from build123d import *

# Parameters (mm, degrees)
F0_W     = 42.8
F0_H     = 42.8
F0_R     = 4.5
F1_DEPTH = 25
F2_R     = 5


with BuildPart() as f1:
    # F0 (on Top) → F1 (new body)
    with BuildSketch(Plane.XY):
        Polygon((24.4, -24.4), (24.4, 24.4), (7.5, 24.4), (-7.5, 24.4), (-24.4, 24.4), (-24.4, -24.4), align=None)
        Rectangle(F0_W, F0_H, mode=Mode.SUBTRACT)
        with BuildLine():
            Line((-7.5, 24.4), (7.5, 24.4))
            Line((7.5, 24.4), (7.5, 36.4))
            ThreePointArc((7.5, 36.4), (0, 28.9), (-7.5, 36.4))
            Line((-7.5, 36.4), (-7.5, 24.4))
        make_face()
        with BuildLine():
            ThreePointArc((-7.5, 36.4), (0, 28.9), (7.5, 36.4))
            ThreePointArc((7.5, 36.4), (0, 43.9), (-7.5, 36.4))
        make_face()
        with Locations((0, 36.4)):
            Circle(F0_R, mode=Mode.SUBTRACT)
    extrude(amount=F1_DEPTH)

    # F2
    f2_edges = [f1.edges().sort_by_distance(p)[0] for p in [
        (7.5, 24.4, 12.5),
        (-7.5, 24.4, 12.5),
    ]]
    fillet(f2_edges, radius=F2_R)


solid = f1.part
Source: CAD feature listing. Evaluate the final solid. Frame: model axes, mm. A direction names the side the tool comes from. Round coordinates to 2 decimals unless told otherwise and drop trailing zeros. Loops run counter-clockwise (first coordinate to the right, second up) from the corner with the lowest first, then second, coordinate; pieces in that order, holes last. Notation, with made-up numbers: (39, 29.25) - (96, 29.25) arc R7 ccw to (96, 42.25) - close; hole circle Ø2 at (79.5, 66). An arc over 180 degrees is marked (long way). Write item = value, one per line. Start each with the question number.
Item 1: Section query B-B on x = 0. Output: boundary loops of the cut face in (y, z), plus the area to 4 significant figures.
Item 2: Mould query, pull axis Y, two halves, no side actions, for faces 1 (the face through (9, 25.83, 12.68)), 2 (the face through (0, 21.4, 12)), 3 (the face through (0, -24.4, 12)). Classes: released by +Y, released by -Y, zero draft, split by the parting line, or undercut.
Item 3: First-contact query: pin 1 Ø1.5 at (y, z) = (30.5, 13) entering from +X; pin 2 Ø2 at (y, z) = (32.5, 12.5) entering from -X; pin 3 Ø3 at (x, z) = (-5.5, 20.5) entering from +Y. Flat tips, straight axial feed; report the tip coordinate or a pass-through.
Item 4: Material intervals for line 1 (Y direction, x = 0, z = 17.5); line 2 (X direction, y = -11.5, z = 22.75), sorted ascending.
Item 5: Reachability of faces 4 (the face through (-7.5, 33, 12)), 5 (the face through (24.4, 0, 12)), 6 (the face through (0.16, 43.9, 12.32)), 7 (the face through (19, 24.4, 12)), 8 (the face through (21.4, 0, 12)) from +Z, -Z, +X, -X, +Y, -Y: full face, straight path, thin tool, end or side. Return the list, or none.
Item 6: Section query C-C on z = 22.5. Output: boundary loops of the cut face in (x, y).
Item 7: Section query A-A on y = 20.5. Output: boundary loops of the cut face in (x, z), plus the area to 3 significant figures.
Results list:
q1.outline = (-24.4, 0) - (-21.4, 0) - (-21.4, 25) - (-24.4, 25) - close; (21.4, 0) - (31.9, 0) - (31.9, 25) - (21.4, 25) - close; (40.9, 0) - (43.9, 0) - (43.9, 25) - (40.9, 25) - close
q1.area = 412.5 mm²
q2.face_1 = released by +Y
q2.face_2 = undercut
q2.face_3 = released by -Y
q3.pin_1 = 7.5
q3.pin_2 = -7.5
q3.pin_3 = 42.74
q4.line_1 = -24.4 to -21.4, 21.4 to 31.9, 40.9 to 43.9
q4.line_2 = -24.4 to -21.4, 21.4 to 24.4
q5.face_4 = +Z, -Z, -X, +Y
q5.face_5 = +Z, -Z, +X, +Y, -Y
q5.face_6 = +Z, -Z, +Y
q5.face_7 = +Z, -Z, +X, +Y
q5.face_8 = +Z, -Z
q6.outline = (-24.4, -24.4) - (24.4, -24.4) - (24.4, 24.4) - (12.5, 24.4) arc R5 cw to (7.5, 29.4) - (7.5, 36.4) arc R7.5 ccw to (-7.5, 36.4) - (-7.5, 29.4) arc R5 cw to (-12.5, 24.4) - (-24.4, 24.4) - close; hole (-21.4, -21.4) - (21.4, -21.4) - (21.4, 21.4) - (-21.4, 21.4) - close; hole circle Ø9 at (0, 36.4)
q7.outline = (-24.4, 0) - (-21.4, 0) - (-21.4, 25) - (-24.4, 25) - close; (21.4, 0) - (24.4, 0) - (24.4, 25) - (21.4, 25) - close
q7.area = 150 mm²
